The model under review builds one solid part; all positions refer to its coordinate system, in mm. A direction names the side the tool comes from. Give positions to 0.01 mm unless a question says otherwise; leave off trailing zeros. Order: outer loops, then holes, each group sorted by start corner. A loop starts at its lowest first (then second) coordinate and runs counter-clockwise, first axis right, second up.
```python
from build123d import *

# Parameters (mm, degrees)
SKETCH2_W                    = 160
SKETCH2_H                    = 60
BASE_FLANGE1_DEPTH           = 4
CUT_EXTRUDE1_DEPTH           = 86.533619121
BREAK_CORNER1_START          = -77.781745931
BREAK_CORNER1_OUTLINE_W      = 114.367532368
BREAK_CORNER1_OUTLINE_H      = 6
BREAK_CORNER1_DEPTH          = 1.414213563
BREAK_CORNER1_START_2        = 33.941125497
BREAK_CORNER1_2_OUTLINE_W    = 1.632467632
BREAK_CORNER1_2_OUTLINE_H    = 6
BREAK_CORNER1_2_DEPTH        = 2.828427125
EDGE_FLANGE1_STRIP_W         = 24
EDGE_FLANGE1_STRIP_H         = 4
EDGE_FLANGE1_STRIP_CUT_DEPTH = 160
EDGE_FLANGE1_DEPTH           = 160
CUT_EXTRUDE2_DEPTH           = 108.944430148
BREAK_CORNER2_START          = -37.830212793
BREAK_CORNER2_OUTLINE_W      = 11.776388924
BREAK_CORNER2_OUTLINE_H      = 7
BREAK_CORNER2_DEPTH          = 10.606601717


# Read off the part's stored shape, not the designer's step: Break-Corner1, Break-Corner2
# Sheet-metal steps are written as plain solids
with BuildPart() as part:
    # Sketch2 → Base-Flange1 (new body)
    with BuildSketch(Plane(origin=(0, 0, 0), x_dir=(1, 0, 0), z_dir=(0, 1, 0))):
        Rectangle(SKETCH2_W, SKETCH2_H)
    extrude(amount=-BASE_FLANGE1_DEPTH)

    # Sketch8 → Cut-Extrude1 (cut, through all)
    with BuildSketch(Plane(origin=(0, 0, 0), x_dir=(1, 0, 0), z_dir=(0, 1, 0))):
        with BuildLine():
            Line((-48, 0), (-48, -31.405477162))
            Line((-48, -31.405477162), (-62, -31.405477162))
            Line((-62, -31.405477162), (-62, 0))
            ThreePointArc((-62, 0), (-55, 7), (-48, 0))
        make_face()
        with BuildLine():
            Line((62, -31.405477162), (62, 0))
            ThreePointArc((62, 0), (55, 7), (48, 0))
            Line((48, 0), (48, -31.405477162))
            Line((48, -31.405477162), (62, -31.405477162))
        make_face()
    extrude(amount=-CUT_EXTRUDE1_DEPTH, mode=Mode.SUBTRACT)

    # Break-Corner1 outline → Break-Corner1 (cut)
    with BuildSketch(Plane(origin=(0, 0, 0), x_dir=(0.707106781186548, 0, 0.707106781186547), z_dir=(0.707106781186547, 0, -0.707106781186548)).offset(BREAK_CORNER1_START)):
        with Locations((19.183766184, 2)):
            Rectangle(BREAK_CORNER1_OUTLINE_W, BREAK_CORNER1_OUTLINE_H)
    extrude(amount=BREAK_CORNER1_DEPTH, mode=Mode.SUBTRACT)

    # Break-Corner1 2 outline → Break-Corner1 2 (cut)
    with BuildSketch(Plane(origin=(0, 0, 0), x_dir=(0.707106781186548, 0, 0.707106781186547), z_dir=(0.707106781186547, 0, -0.707106781186548)).offset(BREAK_CORNER1_START_2)):
        with Locations((77.183766184, 2)):
            Rectangle(BREAK_CORNER1_2_OUTLINE_W, BREAK_CORNER1_2_OUTLINE_H)
    extrude(amount=BREAK_CORNER1_2_DEPTH, mode=Mode.SUBTRACT)

    # Edge-Flange1 strip (across the edge) → Edge-Flange1 strip cut (cut)
    with BuildSketch(Plane(origin=(80, 0, -30), x_dir=(0, 0, 1), z_dir=(-1, 0, 0))):
        with Locations((-4, -2)):
            Rectangle(EDGE_FLANGE1_STRIP_W, EDGE_FLANGE1_STRIP_H)
    extrude(amount=EDGE_FLANGE1_STRIP_CUT_DEPTH, mode=Mode.SUBTRACT)

    # Edge-Flange1 section (across the edge) → Edge-Flange1 (add)
    with BuildSketch(Plane(origin=(80, 0, -30), x_dir=(0, 0, 1), z_dir=(-1, 0, 0))):
        with BuildLine():
            Line((0, 4), (0, 46))
            Line((0, 46), (4, 46))
            Line((4, 46), (4, 4))
            ThreePointArc((4, 4), (5.171572875, 1.171572875), (8, 0))
            Line((8, 0), (8, -4))
            ThreePointArc((8, -4), (2.343145751, -1.656854249), (0, 4))
        make_face()
    extrude(amount=EDGE_FLANGE1_DEPTH)

    # Sketch14 → Cut-Extrude2 (cut, through all)
    with BuildSketch(Plane.XY.offset(-26)):
        with BuildLine():
            Line((5.5, 21), (5.5, 51.754335402))
            Line((5.5, 51.754335402), (-5.5, 51.754335402))
            Line((-5.5, 51.754335402), (-5.5, 21))
            ThreePointArc((-5.5, 21), (0, 15.5), (5.5, 21))
        make_face()
        Polygon((80, 26), (80, 46), (25, 46), align=None)
        Polygon((-80, 26), (-25, 46), (-80, 46), align=None)
    extrude(amount=-CUT_EXTRUDE2_DEPTH, mode=Mode.SUBTRACT)

    # Break-Corner2 outline → Break-Corner2 (cut)
    with BuildSketch(Plane(origin=(0, 0, 0), x_dir=(0.707106781186546, 0.707106781186549, 0), z_dir=(0.707106781186549, -0.707106781186546, 0)).offset(BREAK_CORNER2_START)):
        with Locations((33.111805538, -28.5)):
            Rectangle(BREAK_CORNER2_OUTLINE_W, BREAK_CORNER2_OUTLINE_H)
    extrude(amount=BREAK_CORNER2_DEPTH, mode=Mode.SUBTRACT)


solid = part.part
```
Item 1: For line 1 (X direction, y = -2, z = 12.5); line 2 (Z direction, x = 32.5, y = 24); line 3 (Y direction, x = -63.5, z = 19), list the stretches that pass through material, from the lowest coordinate up.
Values found:
line 1: x = -80 to -62, -48 to 48, 62 to 80
line 2: z = -30 to -26
line 3: y = -4 to 0
Item 2: Take a section at B-B (x = 0). Give the boundary of the cut face in (y, z).
Values found:
outline: (-4, -22) arc R8 ccw to (4, -30) - (15.5, -30) - (15.5, -26) - (4, -26) arc R4 cw to (0, -22) - (0, 30) - (-4, 30) - close
Item 3: Take a section at D-D (x = -55). Give the boundary of the cut face in (y, z).
Values found:
outline: (-4, -22) arc R8 ccw to (4, -30) - (35.09, -30) - (35.09, -26) - (4, -26) arc R4 cw to (0, -22) - (0, -7) - (-4, -7) - close
Item 4: Draft analysis for pull direction X (two halves, no side actions). For faces 6 (the cylindrical face through (1.12, 1.203, -24.859)), 7 (the cylindrical face through (55, -2, -7)), 8 (the flat face through (-80, -1, -7)), state which applies: released by +X, released by -X, zero draft, split by the parting line, or undercut.
Values found:
face 6: zero draft
face 7: undercut
face 8: released by -X
Item 5: Clearance check with flat-ended pins moving along their axes: pin 1 Ø3 at (x, z) = (46.5, -2.5) entering from +Y; pin 2 Ø6 at (x, y) = (-5.5, 4) entering from +Z; pin 3 Ø5 at (x, y) = (-18, 41) entering from +Z. State where each tip first meets the part, or that it passes through.
Values found:
pin 1: stops at y = 0
pin 2: stops at z = -24.65
pin 3: stops at z = -26
Item 6: Take a section at C-C (y = 7). Give the boundary of the cut face in (x, z).
Values found:
outline: (-80, -30) - (80, -30) - (80, -26) - (-80, -26) - close
Item 7: Take a section at A-A (y = 39). Give the boundary of the cut face in (x, z), and give its area (3 significant figures).
Values found:
outline: (-44.25, -30) - (-5.5, -30) - (-5.5, -26) - (-44.25, -26) - close; (5.5, -30) - (44.25, -30) - (44.25, -26) - (5.5, -26) - close
area: 310 mm2
Item 8: For faces 1 (the flat face through (-1, 0, 4)), 2 (the flat face through (70, -2, 30)), 3 (the flat face through (5.5, 32, -28)), 4 (the flat face through (1, 15, -30)), 5 (the flat face through (62, -2, 15)), list the 3-axis set-ups (+Z, -Z, +X, -X, +Y, -Y) from which the entire face can be reached by the end or side of a thin tool; tool diameter is ignored.
Values found:
face 1: +Z, +X, -X, +Y
face 2: +Z, +X, -X, +Y, -Y
face 3: +Z, -Z, +Y
face 4: -Z, +X, -X, +Y, -Y
face 5: +Z, +Y, -Y
